Build history of the part. All positions in model axes, mm. A direction names the side the tool comes from. Coordinates: 2 decimals unless noted, no trailing zeros. Order: outer loops, then holes, each group sorted by start corner. A loop starts at its lowest first (then second) coordinate and runs counter-clockwise, first axis right, second up. Notation, with made-up numbers: (-19, 26.25) - (-12, 26.25) arc R10 ccw to (-12, 44.25) - close; hole circle Ø1 at (0.5, 9.5). An arc over 180 degrees is marked (long way). Write each question's results on one line, items separated by ' | '.
from build123d import *

# Parameters (mm, degrees)
SKETCH2_R           = 12.5
BOSS_EXTRUDE1_DEPTH = 300
SKETCH3_W           = 55
SKETCH3_H           = 70
BOSS_EXTRUDE2_DEPTH = 200
SKETCH4_R           = 5
CUT_EXTRUDE1_DEPTH  = 310.283446049


with BuildPart() as part:
    # Sketch2 → Boss-Extrude1 (new, symmetric)
    with BuildSketch(Plane(origin=(0, 0, 0), x_dir=(0, 0, -1), z_dir=(1, 0, 0))):
        Circle(SKETCH2_R)
    extrude(amount=BOSS_EXTRUDE1_DEPTH, both=True)

    # Sketch3 → Boss-Extrude2 (add, symmetric)
    with BuildSketch(Plane(origin=(0, 0, 0), x_dir=(0, 0, -1), z_dir=(1, 0, 0))):
        with Locations((0, 20)):
            Rectangle(SKETCH3_W, SKETCH3_H)
    extrude(amount=BOSS_EXTRUDE2_DEPTH, both=True)

    # Sketch4 → Cut-Extrude1 (cut, through all)
    with BuildSketch(Plane(origin=(0, 55, 0), x_dir=(1, 0, 0), z_dir=(0, 1, 0))):
        with Locations(Location((150, 0, 0), (0, 0, 270))):
            Circle(SKETCH4_R)
        with Locations(Location((-150, 0, 0), (0, 0, 90))):
            Circle(SKETCH4_R)
    extrude(amount=-CUT_EXTRUDE1_DEPTH, mode=Mode.SUBTRACT)


solid = part.part
1. Probe line 1 (X direction, y = 9, z = 0); line 2 (X direction, y = 37, z = 0); line 3 (Z direction, x = -150, y = 6). List the from-to ranges inside material, lowest first.
Solved:
line 1: x = -300 to -155, -145 to 145, 155 to 300 | line 2: x = -200 to -155, -145 to 145, 155 to 200 | line 3: z = -27.5 to -5, 5 to 27.5
2. Band-saw the part on A-A on x = 150. Give the cut face in (y, z), then the cut area to 3 significant figures.
Solved:
outline: (-15, -27.5) - (55, -27.5) - (55, -5) - (-15, -5) - close; (-15, 5) - (55, 5) - (55, 27.5) - (-15, 27.5) - close | area: 3,150 mm2
3. Band-saw the part on C-C on y = 0. Give the cut face in (x, z).
Solved:
outline: (-300, -12.5) - (-200, -12.5) - (-200, -27.5) - (200, -27.5) - (200, -12.5) - (300, -12.5) - (300, 12.5) - (200, 12.5) - (200, 27.5) - (-200, 27.5) - (-200, 12.5) - (-300, 12.5) - close; hole circle Ø10 at (-150, 0); hole circle Ø10 at (150, 0)
4. Tool access for faces 4 (the face through (-249.3, 3.755, -11.923)), 5 (the face through (145.564, 20.49, 2.307)): list every direction of +Z, -Z, +X, -X, +Y, -Y with a clear straight run to the whole face (end or side of a thin tool).
Solved:
face 4: -X | face 5: +Y, -Y
5. Two-plate mould, pull along Z, no slides. Class faces 1 (the face through (250.7, 3.755, -11.923)), 2 (the face through (-145.564, 20.49, -2.307)), 3 (the face through (3, -15, 0)): +Z half, -Z half, draft (parallel to the pull), parting line (faces both ways), or undercut.
Solved:
face 1: parting line | face 2: undercut | face 3: draft
6. Drop flat-ended pins along their axis: pin 1 Ø4 at (x, z) = (-229.5, -12.5) entering from +Y; pin 2 Ø2 at (y, z) = (29.5, -4) entering from -X; pin 3 Ø2 at (y, z) = (40, -10) entering from +X. Give the stop position or say it passes through.
Solved:
pin 1: stops at y = 6.78 | pin 2: stops at x = -200 | pin 3: stops at x = 200
7. Band-saw the part on B-B on z = 0. Give the cut face in (x, y), then the cut area to 3 significant figures.
Solved:
outline: (-300, -12.5) - (-200, -12.5) - (-200, -15) - (-155, -15) - (-155, 55) - (-200, 55) - (-200, 12.5) - (-300, 12.5) - close; (-145, -15) - (145, -15) - (145, 55) - (-145, 55) - close; (155, -15) - (200, -15) - (200, -12.5) - (300, -12.5) - (300, 12.5) - (200, 12.5) - (200, 55) - (155, 55) - close | area: 31,600 mm2
8. Band-saw the part on D-D on y = 30. Give the cut face in (x, z), then the cut area to 3 significant figures.
Solved:
outline: (-200, -27.5) - (200, -27.5) - (200, 27.5) - (-200, 27.5) - close; hole circle Ø10 at (-150, 0); hole circle Ø10 at (150, 0) | area: 21,800 mm2
